```python
from build123d import *

# Parameters (mm, degrees)
SKETCH1_W           = 125
SKETCH1_H           = 37
BOSS_EXTRUDE1_DEPTH = 3.175
FILLET1_R           = 6
CUT_EXTRUDE1_REACH  = 5.175
SKETCH3_R           = 14.25
SKETCH3_W           = 4.3
SKETCH3_H           = 8.6
SKETCH3_W_2         = 7.5
SKETCH3_H_2         = 13.5
SKETCH6_W           = 20
SKETCH6_H           = 2.5
CUT_EXTRUDE2_DEPTH  = 4.175
FILLET2_R           = 0.5


with BuildPart() as part:
    # Sketch1 → Boss-Extrude1 (new body)
    with BuildSketch(Plane.XY):
        Rectangle(SKETCH1_W, SKETCH1_H)
    extrude(amount=BOSS_EXTRUDE1_DEPTH)

    # Fillet1
    fillet1_edges = [part.edges().sort_by_distance(p)[0] for p in [
        (62.5, -18.5, 1.5875),
        (-62.5, -18.5, 1.5875),
        (-62.5, 18.5, 1.5875),
        (62.5, 18.5, 1.5875),
    ]]
    fillet(fillet1_edges, radius=FILLET1_R)

    # Sketch3 → Cut-Extrude1 (cut, up to next)
    with BuildSketch(Plane.XY.offset(3.175), mode=Mode.PRIVATE) as cut_extrude1_sk1:
        with Locations((42.7653, 1)):
            Circle(SKETCH3_R)
    cut_extrude1_tool1 = extrude(cut_extrude1_sk1.sketch, amount=-CUT_EXTRUDE1_REACH, mode=Mode.PRIVATE) & part.part
    add(cut_extrude1_tool1.solids().sort_by_distance((42.7653, 1, 3.175))[0], mode=Mode.SUBTRACT)
    # Sketch3 → Cut-Extrude1 (cut, up to next)
    with BuildSketch(Plane.XY.offset(3.175), mode=Mode.PRIVATE) as cut_extrude1_sk2:
        with Locations((-42.6527, -1.2074)):
            Circle(SKETCH3_R)
    cut_extrude1_tool2 = extrude(cut_extrude1_sk2.sketch, amount=-CUT_EXTRUDE1_REACH, mode=Mode.PRIVATE) & part.part
    add(cut_extrude1_tool2.solids().sort_by_distance((-42.6527, -1.2074, 3.175))[0], mode=Mode.SUBTRACT)
    # Sketch3 → Cut-Extrude1 (cut, up to next)
    with BuildSketch(Plane.XY.offset(3.175), mode=Mode.PRIVATE) as cut_extrude1_sk3:
        with Locations((0.0563, -1.5037)):
            Rectangle(SKETCH3_W, SKETCH3_H)
    cut_extrude1_tool3 = extrude(cut_extrude1_sk3.sketch, amount=-CUT_EXTRUDE1_REACH, mode=Mode.PRIVATE) & part.part
    add(cut_extrude1_tool3.solids().sort_by_distance((0.0563, -1.5037, 3.175))[0], mode=Mode.SUBTRACT)
    # Sketch3 → Cut-Extrude1 (cut, up to next)
    with BuildSketch(Plane.XY.offset(3.175), mode=Mode.PRIVATE) as cut_extrude1_sk4:
        with Locations((-11.9437, 3.003839217)):
            Rectangle(SKETCH3_W_2, SKETCH3_H_2)
    cut_extrude1_tool4 = extrude(cut_extrude1_sk4.sketch, amount=-CUT_EXTRUDE1_REACH, mode=Mode.PRIVATE) & part.part
    add(cut_extrude1_tool4.solids().sort_by_distance((-11.9437, 3.003839, 3.175))[0], mode=Mode.SUBTRACT)

    # Sketch6 → Cut-Extrude2 (cut, through all)
    with BuildSketch(Plane.XY.offset(3.175)):
        with Locations((27.5, -17.25)):
            Rectangle(SKETCH6_W, SKETCH6_H)
        with Locations((-27.5, -17.25)):
            Rectangle(SKETCH6_W, SKETCH6_H)
        with Locations((-27.5, 17.25)):
            Rectangle(SKETCH6_W, SKETCH6_H)
        with Locations((27.5, 17.25)):
            Rectangle(SKETCH6_W, SKETCH6_H)
    extrude(amount=-CUT_EXTRUDE2_DEPTH, mode=Mode.SUBTRACT)

    # Fillet2
    fillet2_edges = [part.edges().sort_by_distance(p)[0] for p in [
        (-15.6937, -3.746160783, 1.5875),
        (-15.6937, 9.753839217, 1.5875),
        (-8.1937, 9.753839217, 1.5875),
        (-8.1937, -3.746160783, 1.5875),
        (2.2063, 2.7963, 1.5875),
        (2.2063, -5.8037, 1.5875),
        (-2.0937, -5.8037, 1.5875),
        (-2.0937, 2.7963, 1.5875),
    ]]
    fillet(fillet2_edges, radius=FILLET2_R)


solid = part.part
```
The model under review builds one solid part; all positions refer to its coordinate system, in mm. A direction names the side the tool comes from. Round coordinates to 2 decimals unless told otherwise and drop trailing zeros. Loops run counter-clockwise (first coordinate to the right, second up) from the corner with the lowest first, then second, coordinate; pieces in that order, holes last. Notation, with made-up numbers: M 52,8.25 L 109,8.25 A24 cw 109,22.25 Z; hole C 13.5,50.5 d10. An arc over 180 degrees is marked long. Answer as a JSON object with one key per item and string values.
(1) Take a section at C-C on y = -11. Give the boundary of the cut face in (x, z) (3 decimals), and give its area (3 significant figures).
Resolved:
{"outline": "M -62.5,0 L -53.005,0 L -53.005,3.175 L -62.5,3.175 Z; M -32.301,0 L 35.08,0 L 35.08,3.175 L -32.301,3.175 Z; M 50.451,0 L 62.5,0 L 62.5,3.175 L 50.451,3.175 Z", "area": "282 mm²"}
(2) Take a section at A-A on y = 1. Give the boundary of the cut face in (x, z) (3 decimals).
Resolved:
{"outline": "M -62.5,0 L -56.731,0 L -56.731,3.175 L -62.5,3.175 Z; M -28.575,0 L -15.694,0 L -15.694,3.175 L -28.575,3.175 Z; M -8.194,0 L -2.094,0 L -2.094,3.175 L -8.194,3.175 Z; M 2.206,0 L 28.515,0 L 28.515,3.175 L 2.206,3.175 Z; M 57.015,0 L 62.5,0 L 62.5,3.175 L 57.015,3.175 Z"}
(3) Take a section at B-B on x = -50. Give the boundary of the cut face in (y, z) (3 decimals), and give its area (3 significant figures).
Resolved:
{"outline": "M -18.5,0 L -13.417,0 L -13.417,3.175 L -18.5,3.175 Z; M 11.002,0 L 18.5,0 L 18.5,3.175 L 11.002,3.175 Z", "area": "39.9 mm²"}
(4) Take a section at D-D on x = 46. Give the boundary of the cut face in (y, z) (3 decimals).
Resolved:
{"outline": "M -18.5,0 L -12.878,0 L -12.878,3.175 L -18.5,3.175 Z; M 14.878,0 L 18.5,0 L 18.5,3.175 L 14.878,3.175 Z"}
(5) Draft analysis for pull direction Y (two halves, no side actions). For faces 4 (the cylindrical face through (-60.789, -16.696, 1.61)), 5 (the flat face through (-12, 9.754, 2)), 6 (the flat face through (62.5, 0, 2)), state which applies: released by +Y, released by -Y, zero draft, split by the parting line, or undercut.
Resolved:
{"face 4": "released by -Y", "face 5": "undercut", "face 6": "zero draft"}
(6) Clearance check with flat-ended pins moving along their axes: P1, Ø0.8, axis at y = -16.5, z = 1.5, coming from the -X side; P2, Ø17, axis at x = 42.77, y = 1, coming from the -Z side; P3, Ø1, axis at x = -29.5, z = 2.5, coming from the -Y side. State where each tip first meets the part, or that it passes through.
Resolved:
{"P1": "x = -61.3", "P2": "through", "P3": "y = -16"}
(7) Tool access review of faces 1 (the flat face through (-8.194, 3, 2)), 2 (the flat face through (-37.5, -17, 2)), 3 (the flat face through (37.5, 17, 2)): name each direction out of +Z, -Z, +X, -X, +Y, -Y from which nothing blocks a thin tool from reaching the whole face with its end or side.
Resolved:
{"face 1": "+Z, -Z", "face 2": "+Z, -Z, -Y", "face 3": "+Z, -Z, +Y"}
(8) To check wall thickness, follow line 1 along X through (y, z) = (-5.5, 0.3); line 2 along X through (y, z) = (-1, 0.95); line 3 along X through (y, z) = (1.5, 0.35). State the ranges of each line that lie inside material, in increasing order.
Resolved:
{"line 1": "-62.5 to -56.24, -29.06 to -2.05, 2.17 to 30.08, 55.45 to 62.5", "line 2": "-62.5 to -56.9, -28.4 to -15.69, -8.19 to -2.09, 2.21 to 28.66, 56.87 to 62.5", "line 3": "-62.5 to -56.64, -28.66 to -15.69, -8.19 to -2.09, 2.21 to 28.52, 57.01 to 62.5"}
